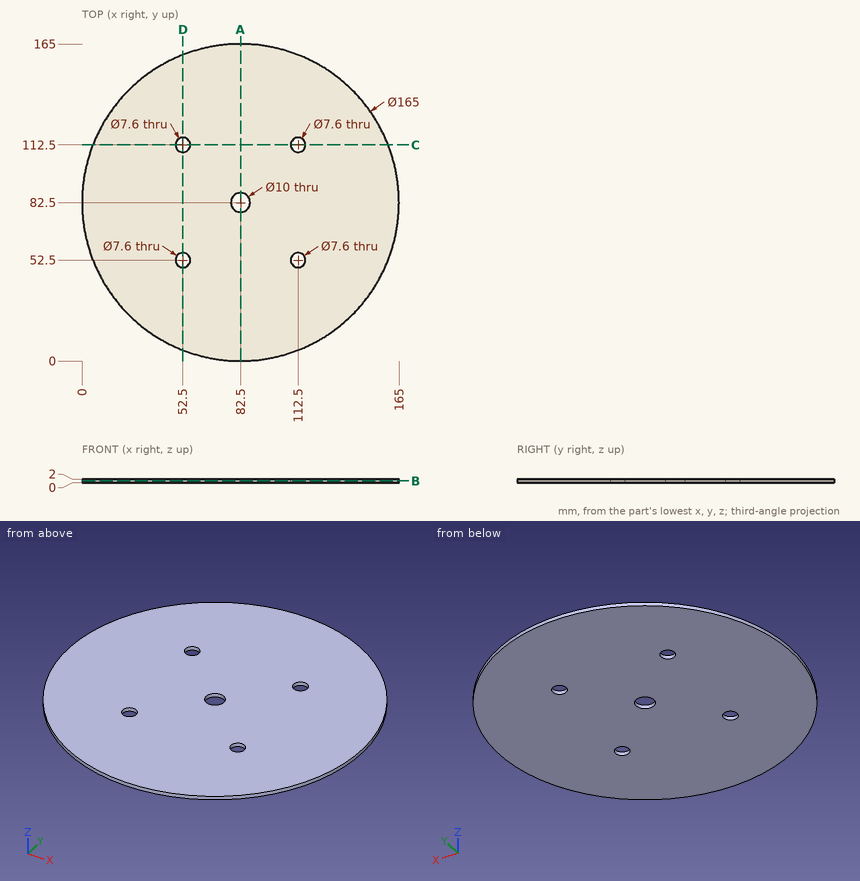
For this review, use the dimensioned drawing (mm, ordinates from the lowest corner) and the shaded views. Coordinates: 2 decimals unless noted, no trailing zeros. Write each loop counter-clockwise with the first axis right and the second up, starting at its lowest first coordinate (ties: lowest second). Pieces come first, ordered by that corner, then holes. Notation, with made-up numbers: (7.5, 21.5) - (45.5, 21.5) arc R10 ccw to (45.5, 26.5) - close; hole circle Ø5 at (31, -38). An arc over 180 degrees is marked (long way). Answer in a Markdown table with one row per item. Add a question column.
Q1. Consider section C-C on y = 112.5. Give the boundary of the cut face in (x, z).
Q2. Consider section A-A on x = 82.5. Give the boundary of the cut face in (y, z), then the cut area to 3 significant figures.
Q3. Consider section B-B on z = 1. Give the boundary of the cut face in (x, y), then the cut area to 3 significant figures.
Q4. To check wall thickness, follow line 1 along Y through (x, z) = (112.5, 1.5); line 2 along Y through (x, z) = (55, 1.7); line 3 along Y through (x, z) = (79, 1.6). State the ranges of each line that lie inside material, in increasing order. Write a range as from..to.
Answers below:
| question | item | result |
|---|---|---|
| 1 | outline | (5.65, 0) - (48.7, 0) - (48.7, 2) - (5.65, 2) - close; (56.3, 0) - (108.7, 0) - (108.7, 2) - (56.3, 2) - close; (116.3, 0) - (159.35, 0) - (159.35, 2) - (116.3, 2) - close |
| 2 | outline | (0, 0) - (77.5, 0) - (77.5, 2) - (0, 2) - close; (87.5, 0) - (165, 0) - (165, 2) - (87.5, 2) - close |
| 2 | area | 310 mm² |
| 3 | outline | circle Ø165 at (82.5, 82.5); hole circle Ø7.6 at (52.5, 52.5); hole circle Ø7.6 at (52.5, 112.5); hole circle Ø10 at (82.5, 82.5); hole circle Ø7.6 at (112.5, 52.5); hole circle Ø7.6 at (112.5, 112.5) |
| 3 | area | 21,100 mm² |
| 4 | line 1 | 5.65..48.7, 56.3..108.7, 116.3..159.35 |
| 4 | line 2 | 4.72..49.64, 55.36..109.64, 115.36..160.28 |
| 4 | line 3 | 0.07..78.93, 86.07..164.93 |
